from build123d import *

# Parameters (mm, degrees)
SKETCH1_W           = 81
SKETCH1_H           = 116
BOSS_EXTRUDE1_DEPTH = 3
CUT_EXTRUDE2_DEPTH  = 81
CUT_EXTRUDE3_DEPTH  = 81
SKETCH6_W           = 1.85
SKETCH6_H           = 1.55
CUT_EXTRUDE5_DEPTH  = 0.6
FILLET6_R           = 0.4
CHAMFER2_SIZE       = 0.2
SKETCH7_W           = 1.85
SKETCH7_H           = 1.55
CUT_EXTRUDE6_DEPTH  = 0.6
FILLET7_R           = 0.4
CHAMFER3_SIZE       = 0.2
SKETCH10_W          = 81
SKETCH10_H          = 113.1
CUT_EXTRUDE7_DEPTH  = 0.2
FILLET8_R           = 0.4
BOSS_EXTRUDE2_DEPTH = 3
FILLET10_R          = 0.5
CUT_EXTRUDE8_REACH  = 142.423
SKETCH11_W          = 113.1
SKETCH11_H          = 0.1


with BuildPart() as part:
    # Sketch1 → Boss-Extrude1 (new body)
    with BuildSketch(Plane(origin=(0, 0, 0), x_dir=(1, 0, 0), z_dir=(0, 1, 0))):
        with Locations((40.5, 58)):
            Rectangle(SKETCH1_W, SKETCH1_H)
    extrude(amount=BOSS_EXTRUDE1_DEPTH)

    # Sketch2 → Cut-Extrude2 (cut)
    with BuildSketch(Plane(origin=(81, 0, 0), x_dir=(0, 0, -1), z_dir=(1, 0, 0))):
        Polygon((0, 3), (3, 3), (3, 1.75), (1.25, 1.75), (1.25, 0), (0, 0), align=None)
        Polygon((114.75, 0), (116, 0), (116, 3), (113, 3), (113, 1.75), (114.75, 1.75), align=None)
    extrude(amount=-CUT_EXTRUDE2_DEPTH, mode=Mode.SUBTRACT)

    # Sketch4 → Cut-Extrude3 (cut)
    with BuildSketch(Plane(origin=(81, 0, 0), x_dir=(0, 0, -1), z_dir=(1, 0, 0))):
        Polygon((3.2, 3), (3, 3), (3, 1.75), (1.25, 1.75), (1.25, 0), (1.45, 0), (1.45, 1.55), (3.2, 1.55), align=None)
        Polygon((114.75, 0), (114.55, 0), (114.55, 1.55), (112.8, 1.55), (112.8, 3), (113, 3), (113, 1.75), (114.75, 1.75), align=None)
    extrude(amount=-CUT_EXTRUDE3_DEPTH, mode=Mode.SUBTRACT)

    # Sketch6 → Cut-Extrude5 (cut)
    with BuildSketch(Plane.XY.offset(-1.45)):
        with Locations((3, 0.775)):
            Rectangle(SKETCH6_W, SKETCH6_H)
    extrude(amount=-CUT_EXTRUDE5_DEPTH, mode=Mode.SUBTRACT)

    # Fillet6
    fillet6_edges = [part.edges().sort_by_distance(p)[0] for p in [
        (2.075, 0.775, -1.45),
    ]]
    fillet(fillet6_edges, radius=FILLET6_R)

    # Chamfer2
    chamfer2_edges = [part.edges().sort_by_distance(p)[0] for p in [
        (3.925, 0.775, -1.45),
    ]]
    chamfer(chamfer2_edges, length=CHAMFER2_SIZE)

    # Sketch7 → Cut-Extrude6 (cut)
    with BuildSketch(Plane(origin=(0, 0, -114.55), x_dir=(-1, 0, 0), z_dir=(0, 0, -1))):
        with Locations((-3, 0.775)):
            Rectangle(SKETCH7_W, SKETCH7_H)
    extrude(amount=-CUT_EXTRUDE6_DEPTH, mode=Mode.SUBTRACT)

    # Fillet7
    fillet7_edges = [part.edges().sort_by_distance(p)[0] for p in [
        (2.075, 0.775, -114.55),
    ]]
    fillet(fillet7_edges, radius=FILLET7_R)

    # Chamfer3
    chamfer3_edges = [part.edges().sort_by_distance(p)[0] for p in [
        (3.925, 0.775, -114.55),
    ]]
    chamfer(chamfer3_edges, length=CHAMFER3_SIZE)

    # Sketch10 → Cut-Extrude7 (cut)
    with BuildSketch(Plane(origin=(0, 0, 0), x_dir=(-1, 0, 0), z_dir=(0, -1, 0))):
        with Locations((-40.5, 58)):
            Rectangle(SKETCH10_W, SKETCH10_H)
    extrude(amount=-CUT_EXTRUDE7_DEPTH, mode=Mode.SUBTRACT)

    # Fillet8
    fillet8_edges = [part.edges().sort_by_distance(p)[0] for p in [
        (0, 0.875, -114.55),
        (0, 0.875, -1.45),
    ]]
    fillet(fillet8_edges, radius=FILLET8_R)

    # Sketch9 → Boss-Extrude2 (add)
    with BuildSketch(Plane(origin=(0, 3, 0), x_dir=(1, 0, 0), z_dir=(0, 1, 0))):
        with BuildLine():
            Line((74.5, 38), (74.5, 78))
            ThreePointArc((74.5, 78), (76, 79.5), (77.5, 78))
            Line((77.5, 78), (77.5, 38))
            ThreePointArc((77.5, 38), (76, 36.5), (74.5, 38))
        make_face()
    extrude(amount=BOSS_EXTRUDE2_DEPTH)

    # Fillet10
    fillet10_edges = [part.edges().sort_by_distance(p)[0] for p in [
        (76, 3, -36.5),
        (77.5, 3, -58),
        (76, 3, -79.5),
        (74.5, 3, -58),
        (76, 6, -36.5),
        (77.5, 6, -58),
        (76, 6, -79.5),
        (74.5, 6, -58),
    ]]
    fillet(fillet10_edges, radius=FILLET10_R)

    # Cut-Extrude8: up to this face of the body (flat: up to its plane)
    cut_extrude8_end = Plane(part.part.faces().sort_by_distance((0, 1.591489816, -58))[0])
    # Sketch11 → Cut-Extrude8 (cut, up to the picked face)
    with BuildSketch(Plane(origin=(81, 0, 0), x_dir=(0, 0, -1), z_dir=(1, 0, 0)), mode=Mode.PRIVATE) as cut_extrude8_sk1:
        with Locations((58, 0.25)):
            Rectangle(SKETCH11_W, SKETCH11_H)
    cut_extrude8_tool1 = split(extrude(cut_extrude8_sk1.sketch, amount=-CUT_EXTRUDE8_REACH, mode=Mode.PRIVATE), bisect_by=cut_extrude8_end, keep=Keep.BOTH, mode=Mode.PRIVATE)
    add(cut_extrude8_tool1.solids().sort_by(Axis((81, 0.25, -58), (-1, 0, 0)))[0], mode=Mode.SUBTRACT)


solid = part.part
Design review of the part built by this model. Coordinates are the model's own, in mm. Coordinates: 2 decimals unless noted, no trailing zeros. Order: outer loops, then holes, each group sorted by start corner. A loop starts at its lowest first (then second) coordinate and runs counter-clockwise, first axis right, second up.
Item 1: For pin 1 Ø1.9 at (x, z) = (53, -2.5) entering from +Y; pin 2 Ø0.6 at (y, z) = (5, -51) entering from +X; pin 3 Ø1.6 at (y, z) = (4, -61.5) entering from -X, all flat-tipped, find the tip position at first contact; note any pin that passes through.
Item 2: Take a section at C-C, the plane z = -29. Write out the cut boundary in (x, y), then the cut area to 3 significant figures.
Item 3: For line 1 (Y direction, x = 45, z = -98.5); line 2 (Z direction, x = 13, y = 2); line 3 (X direction, y = 5.65, z = -56), list the stretches that pass through material, from the lowest coordinate up.
Item 4: Take a section at A-A, the plane x = 43. Write out the cut boundary in (y, z).
Item 5: Take a section at B-B, the plane z = -46. Write out the cut boundary in (x, y).
The answers:
1. pin 1: stops at y = 3
1. pin 2: stops at x = 77.5
1. pin 3: stops at x = 74.4
2. outline: (0, 0.3) - (81, 0.3) - (81, 3) - (0, 3) - close
2. area: 219 mm2
3. line 1: y = 0.3 to 3
3. line 2: z = -112.8 to -3.2
3. line 3: x = 74.52 to 77.48
4. outline: (0.3, -114.55) - (1.55, -114.55) - (1.55, -112.8) - (3, -112.8) - (3, -3.2) - (1.55, -3.2) - (1.55, -1.45) - (0.3, -1.45) - close
5. outline: (0, 0.3) - (81, 0.3) - (81, 3) - (78, 3) arc R0.5 cw to (77.5, 3.5) - (77.5, 5.5) arc R0.5 ccw to (77, 6) - (75, 6) arc R0.5 ccw to (74.5, 5.5) - (74.5, 3.5) arc R0.5 cw to (74, 3) - (0, 3) - close
